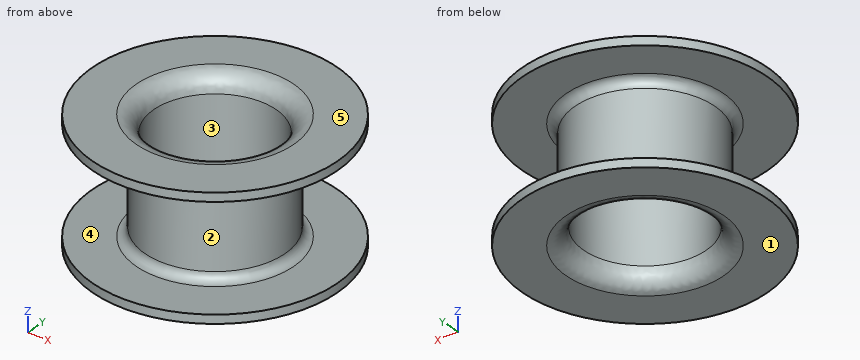
from build123d import *
from build123d.topology import SkipClean

# Parameters (mm, degrees)
SKETCH_1_R      = 3.5
SKETCH_1_R_2    = 1.75
EXTRUDE_1_DEPTH = 0.25
EXTRUDE_START   = 3
SKETCH_2_R      = 2
SKETCH_2_R_2    = 1.75
EXTRUDE_2_DEPTH = 3
EXTRUDE_START_2 = 0.25
SKETCH_3_R      = 3.5
SKETCH_3_R_2    = 1.75
EXTRUDE_3_DEPTH = 0.25
FILLET_1_R      = 0.25
FILLET_2_R      = 0.5


with BuildPart() as part:
    # Эскиз1 → Вытянуть1 (new body)
    with BuildSketch(Plane.XY):
        Circle(SKETCH_1_R)
        Circle(SKETCH_1_R_2, mode=Mode.SUBTRACT)
    extrude(amount=EXTRUDE_1_DEPTH)

    # Эскиз2 → Вытянуть2 (add)
    with SkipClean():  # the faces are left unmerged after this step: merging them gives an invalid solid
        with BuildSketch(Plane(origin=(0, 0, 0), x_dir=(-1, 0, 0), z_dir=(0, 0, -1)).offset(EXTRUDE_START)):
            with Locations(Location((0, 0, 0), (0, 0, 180))):
                Circle(SKETCH_2_R)
            Circle(SKETCH_2_R_2, mode=Mode.SUBTRACT)
        extrude(amount=-EXTRUDE_2_DEPTH)

    # Эскиз3 → Вытянуть3 (add)
    with SkipClean():  # the faces are left unmerged after this step: merging them gives an invalid solid
        with BuildSketch(Plane(origin=(0, 0, -3), x_dir=(-1, 0, 0), z_dir=(0, 0, -1)).offset(EXTRUDE_START_2)):
            with Locations(Location((0, 0, 0), (0, 0, 180))):
                Circle(SKETCH_3_R)
            Circle(SKETCH_3_R_2, mode=Mode.SUBTRACT)
        extrude(amount=-EXTRUDE_3_DEPTH)

    # Скругление1
    fillet_1_edges = [part.edges().sort_by_distance(p)[0] for p in [
        (-2, 0, -3),
        (-2, 0, 0),
    ]]
    fillet(fillet_1_edges, radius=FILLET_1_R)

    # Скругление2
    fillet_2_edges = [part.edges().sort_by_distance(p)[0] for p in [
        (1.75, 0, -3.25),
        (-1.75, 0, 0.25),
    ]]
    fillet(fillet_2_edges, radius=FILLET_2_R)


solid = part.part
Geometry check sheet. Reference: the model listing, model coordinates, mm. Face numbers are marked on the shaded views. A direction names the side the tool comes from. Round coordinates to 2 decimals unless told otherwise and drop trailing zeros. Order: outer loops, then holes, each group sorted by start corner. A loop starts at its lowest first (then second) coordinate and runs counter-clockwise, first axis right, second up. Notation, with made-up numbers: (-25, 8) - (29, 8) arc R22 ccw to (29, 25) - close; hole circle Ø2 at (18, 81.25). An arc over 180 degrees is marked (long way). One line per question, with ' | ' between items. Start each with the question number.
(1) Sectioned sample at C-C on z = -1.05. Record the cut outline in (x, y), and give its area (3 significant figures).
(2) Sectioned sample at A-A on x = 3. Record the cut outline in (y, z).
(3) Depth check by flat-ended pin: pin 1 Ø3 at (x, y) = (0, 0) entering from -Z. Enter the tip coordinate at first touch or a pass-through.
(4) Release check for a two-part mould opening along X. For the marked faces 1, 2 and 3 record: released by +X, released by -X, zero draft, split by the parting line, or undercut.
(5) Sectioned sample at B-B on y = 2.75. Record the cut outline in (x, z).
(6) Access from +Z, -Z, +X, -X, +Y, -Y to the whole of each face (thin tool, end or side, straight path). Record for the marked faces 4 and 5.
(7) Thickness scan on L1, parallel to Z at x = -2.25, y = 1.25; L2, parallel to Y at x = 0, z = -1.45. Record the ranges inside material, lowest first. Write a range as [from, to].
Conclusion:
1) outline: circle Ø4 at (0, 0); hole circle Ø3.5 at (0, 0) | area: 2.95 mm2
2) outline: (-1.8, -3.25) - (1.8, -3.25) - (1.8, -3) - (-1.8, -3) - close; (-1.8, 0) - (1.8, 0) - (1.8, 0.25) - (-1.8, 0.25) - close
3) pin 1: passes through
4) face 1: zero draft | face 2: split by the parting line | face 3: undercut
5) outline: (-2.17, -3.25) - (2.17, -3.25) - (2.17, -3) - (-2.17, -3) - close; (-2.17, 0) - (2.17, 0) - (2.17, 0.25) - (-2.17, 0.25) - close
6) face 4: none | face 5: +Z, +X, -X, +Y, -Y
7) L1: z = [-3.25, -3], [0, 0.25] | L2: y = [-2, -1.75], [1.75, 2]
